```python
from build123d import *

# Parameters (mm, degrees)
BOSS_EXTRUDE1_DEPTH      = 22
BOSS_EXTRUDE1_DEPTH_BACK = 22
CUT_EXTRUDE1_DEPTH       = 12
CUT_EXTRUDE1_DEPTH_BACK  = 12
BOSS_EXTRUDE2_DEPTH      = 22
BOSS_EXTRUDE2_DEPTH_BACK = 22
SKETCH1_4_R              = 19
SKETCH2_W                = 20
SKETCH2_H                = 71.319649742
CUT_EXTRUDE2_DEPTH       = 134.379158792


with BuildPart() as part:
    # Sketch1 → Boss-Extrude1 (new, two sides: drawn at the far end of the back side and taken through both)
    with BuildSketch(Plane.XY.offset(-BOSS_EXTRUDE1_DEPTH_BACK)):
        Polygon((-30, 11), (-65, -11), (-14, -11), (-23, 4), (23, 4), (14, -11), (65, -11), (30, 11), align=None)
        Polygon((65, 11), (30, 11), (65, -11), align=None)
        Polygon((-65, 11), (-65, -11), (-30, 11), align=None)
    extrude(amount=BOSS_EXTRUDE1_DEPTH + BOSS_EXTRUDE1_DEPTH_BACK)

    # Sketch1_3 → Cut-Extrude1 (cut, two sides: drawn at the far end of the back side and taken through both)
    with BuildSketch(Plane.XY.offset(-CUT_EXTRUDE1_DEPTH_BACK)):
        Polygon((-65, 11), (-65, -11), (-30, 11), align=None)
        Polygon((65, 11), (30, 11), (65, -11), align=None)
    extrude(amount=CUT_EXTRUDE1_DEPTH + CUT_EXTRUDE1_DEPTH_BACK, mode=Mode.SUBTRACT)

    # Sketch1_4 → Boss-Extrude2 (add, two sides: drawn at the far end of the back side and taken through both)
    with BuildSketch(Plane.XY.offset(-BOSS_EXTRUDE2_DEPTH_BACK)):
        with BuildLine():
            Line((-30, 61), (-30, 11))
            Line((-30, 11), (30, 11))
            Line((30, 11), (30, 61))
            ThreePointArc((30, 61), (0, 91), (-30, 61))
        make_face()
        with Locations((0, 61)):
            Circle(SKETCH1_4_R, mode=Mode.SUBTRACT)
    extrude(amount=BOSS_EXTRUDE2_DEPTH + BOSS_EXTRUDE2_DEPTH_BACK)

    # Sketch2 → Cut-Extrude2 (cut, through all)
    with BuildSketch(Plane(origin=(30, 0, 0), x_dir=(0, 0, -1), z_dir=(1, 0, 0))):
        with Locations((0, 61.659824871)):
            Rectangle(SKETCH2_W, SKETCH2_H)
    extrude(amount=-CUT_EXTRUDE2_DEPTH, mode=Mode.SUBTRACT)


solid = part.part
```
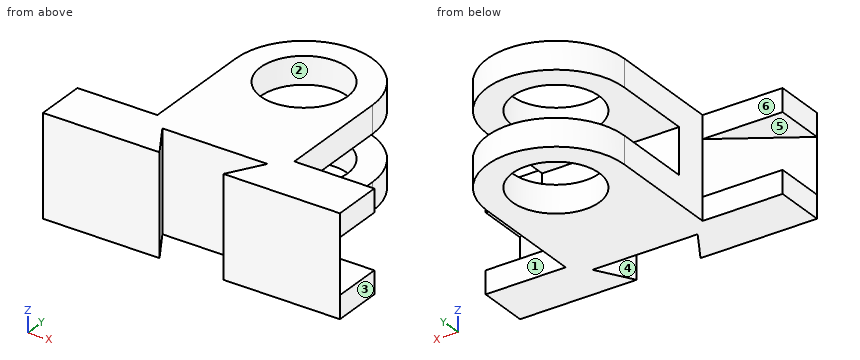
The model under review builds one solid part; all positions refer to its coordinate system, in mm. Face numbers are marked on the shaded views. A direction names the side the tool comes from. Round coordinates to 2 decimals unless told otherwise and drop trailing zeros. Loops run counter-clockwise (first coordinate to the right, second up) from the corner with the lowest first, then second, coordinate; pieces in that order, holes last.
Item 1: For the marked faces 4, 5 and 6, list the 3-axis set-ups (+Z, -Z, +X, -X, +Y, -Y) from which the entire face can be reached by the end or side of a thin tool; tool diameter is ignored.
Determined:
face 4: +Z, -Z
face 5: -X, +Y
face 6: +Z, -Z, -X, +Y
Item 2: Take a section at C-C (x = 0). Write out the cut boundary in (y, z), then the cut area to 3 significant figures.
Determined:
outline: (4, -22) - (42, -22) - (42, -10) - (26, -10) - (26, 10) - (42, 10) - (42, 22) - (4, 22) - close; (80, -22) - (91, -22) - (91, -10) - (80, -10) - close; (80, 10) - (91, 10) - (91, 22) - (80, 22) - close
area: 1,620 mm2
Item 3: Mouldability with a two-part tool opening along Y and no side actions: class the marked faces 1, 2 and 3 as released by +Y, released by -Y, zero draft, split by the parting line, or undercut.
Determined:
face 1: released by +Y
face 2: undercut
face 3: zero draft
Item 4: Clearance check with flat-ended pins moving along their axes: pin 1 Ø22 at (x, z) = (-4, -2.5) entering from +Y; pin 2 Ø3 at (x, z) = (-53, -15) entering from +Y; pin 3 Ø2 at (x, z) = (25.5, 11.5) entering from +Y. State where each tip first meets the part, or that it passes through.
Determined:
pin 1: stops at y = 91
pin 2: stops at y = 11
pin 3: stops at y = 78.31
Item 5: Take a section at A-A (y = 30). Write out the cut boundary in (x, z).
Determined:
outline: (-30, -22) - (30, -22) - (30, -10) - (-30, -10) - close; (-30, 10) - (30, 10) - (30, 22) - (-30, 22) - close
Item 6: Take a section at B-B (z = -15). Write out the cut boundary in (x, y).
Determined:
outline: (-65, -11) - (-14, -11) - (-23, 4) - (23, 4) - (14, -11) - (65, -11) - (65, 11) - (30, 11) - (30, 61) arc R30 ccw to (-30, 61) - (-30, 11) - (-65, 11) - close; hole circle Ø38 at (0, 61)
Item 7: Take a section at D-D (y = 74.5). Write out the cut boundary in (x, z).
Determined:
outline: (-26.79, -22) - (-13.37, -22) - (-13.37, -10) - (-26.79, -10) - close; (-26.79, 10) - (-13.37, 10) - (-13.37, 22) - (-26.79, 22) - close; (13.37, -22) - (26.79, -22) - (26.79, -10) - (13.37, -10) - close; (13.37, 10) - (26.79, 10) - (26.79, 22) - (13.37, 22) - close
Item 8: For line 1 (Z direction, x = -42, y = 6.5); line 2 (Z direction, x = 23, y = 35.5); line 3 (Y direction, x = 0, z = -14.75), list the stretches that pass through material, from the lowest coordinate up.
Determined:
line 1: z = -22 to -12, 12 to 22
line 2: z = -22 to -10, 10 to 22
line 3: y = 4 to 42, 80 to 91
